```python
from build123d import *

# Parameters (mm, degrees)
SKETCH1_W                = 5.5
SKETCH1_H                = 14.5
SKETCH1_R                = 0.4064
BOSS_EXTRUDE1_DEPTH      = 1.75
FILLET1_R                = 2.5
CIRPATTERN1_COUNT        = 4
FILLET1_OF_CIRPATTERN1_R = 2.5
CUT_EXTRUDE1_REACH       = 22.581
SKETCH2_R                = 1


with BuildPart() as part:
    # Sketch1 → Boss-Extrude1 (new body)
    with BuildSketch(Plane(origin=(0, 0, 0), x_dir=(1, 0, 0), z_dir=(0, 1, 0))):
        with Locations((0, 7.25)):
            Rectangle(SKETCH1_W, SKETCH1_H)
        with Locations(Location((0, 12, 0), (0, 0, 270))):
            Circle(SKETCH1_R, mode=Mode.SUBTRACT)
        with Locations(Location((0, 10, 0), (0, 0, 270))):
            Circle(SKETCH1_R, mode=Mode.SUBTRACT)
        with Locations(Location((0, 8, 0), (0, 0, 270))):
            Circle(SKETCH1_R, mode=Mode.SUBTRACT)
        with Locations(Location((0, 6, 0), (0, 0, 270))):
            Circle(SKETCH1_R, mode=Mode.SUBTRACT)
    boss_extrude1 = extrude(amount=BOSS_EXTRUDE1_DEPTH)

    # Fillet1
    fillet1_edges = [part.edges().sort_by_distance(p)[0] for p in [
        (-2.75, 0.875, -14.5),
        (2.75, 0.875, -14.5),
    ]]
    fillet(fillet1_edges, radius=FILLET1_R)

    # CirPattern1: Boss-Extrude1 ×4 about axis
    cirpattern1_axis = Axis((0, 0, 0), (0, 1, 0))
    for i in range(1, CIRPATTERN1_COUNT):
        add(boss_extrude1.rotate(cirpattern1_axis, i * 360 / CIRPATTERN1_COUNT))

    # Fillet1 of CirPattern1
    fillet1_of_cirpattern1_edges = [part.edges().sort_by_distance(p)[0] for p in [
        (-14.5, 0.875, 2.75),
        (-14.5, 0.875, -2.75),
        (2.75, 0.875, 14.5),
        (-2.75, 0.875, 14.5),
        (14.5, 0.875, -2.75),
        (14.5, 0.875, 2.75),
    ]]
    fillet(fillet1_of_cirpattern1_edges, radius=FILLET1_OF_CIRPATTERN1_R)

    # Sketch2 → Cut-Extrude1 (cut, up to next)
    with BuildSketch(Plane(origin=(0, 1.75, 0), x_dir=(1, 0, 0), z_dir=(0, 1, 0)), mode=Mode.PRIVATE) as cut_extrude1_sk1:
        with Locations(Location((0, 0, 0), (0, 0, 270))):
            Circle(SKETCH2_R)
    cut_extrude1_tool1 = extrude(cut_extrude1_sk1.sketch, amount=-CUT_EXTRUDE1_REACH, mode=Mode.PRIVATE) & part.part
    add(cut_extrude1_tool1.solids().sort_by_distance((0, 1.75, 0))[0], mode=Mode.SUBTRACT)


solid = part.part
```
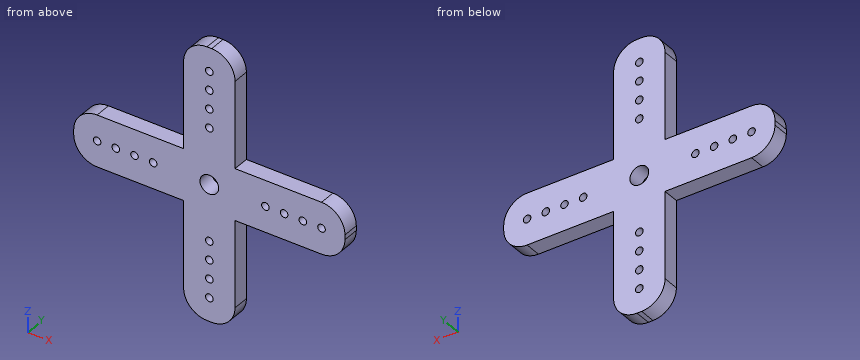
The model under review builds one solid part; all positions refer to its coordinate system, in mm. Give positions to 0.01 mm unless a question says otherwise; leave off trailing zeros. Write each loop counter-clockwise with the first axis right and the second up, starting at its lowest first coordinate (ties: lowest second). Pieces come first, ordered by that corner, then holes. Notation, with made-up numbers: (57, -28.5) -> (108, -28.5) arc R11 ccw to (108, -16.5) -> close; hole circle Ø4 at (-2, 8). An arc over 180 degrees is marked (long way). Answer in a Markdown table with one row per item.
1) Add section B-B on z = -8. State the section outline as (x, y) points.
Worked answers:
| item | result |
|---|---|
| outline | (-2.75, 0) -> (-0.41, 0) -> (-0.41, 1.75) -> (-2.75, 1.75) -> close; (0.41, 0) -> (2.75, 0) -> (2.75, 1.75) -> (0.41, 1.75) -> close |
2) Add section C-C on x = -11.25. State the section outline as (y, z) points, plus the area to 4 significant figures.
Worked answers:
| item | result |
|---|---|
| outline | (0, -2.75) -> (1.75, -2.75) -> (1.75, 2.75) -> (0, 2.75) -> close |
| area | 9.625 mm² |
3) Add section A-A on x = 6. State the section outline as (y, z) points.
Worked answers:
| item | result |
|---|---|
| outline | (0, -2.75) -> (1.75, -2.75) -> (1.75, -0.41) -> (0, -0.41) -> close; (0, 0.41) -> (1.75, 0.41) -> (1.75, 2.75) -> (0, 2.75) -> close |
4) For L1, parallel to X at y = 0.7, z = -6, list the stretches that pass through material, from the lowest coordinate up. Write a range as [from, to].
Worked answers:
| item | result |
|---|---|
| L1 | [-2.75, -0.41], [0.41, 2.75] |
5) Add section D-D on y = 0.95. Count the separate pieces of the cut face and the enclosed holes in it, plus the area to 3 significant figures.
Worked answers:
| item | result |
|---|---|
| separate pieces | 1 |
| enclosed holes | 17 |
| area | 267 mm² |
6) Clearance check with flat-ended pins moving along their axes: P1, Ø0.5, axis at y = 1, z = -7, coming from the -X side; P2, Ø0.5, axis at x = -6.5, y = 1, coming from the +Z side; P3, Ø0.9, axis at x = 6, y = 1, coming from the -Z side. State where each tip first meets the part, or that it passes through.
Worked answers:
| item | result |
|---|---|
| P1 | x = -2.75 |
| P2 | z = 2.75 |
| P3 | z = -2.75 |
